Build history of the part. All positions in model axes, mm. Face numbers are marked on the shaded views. A direction names the side the tool comes from. Coordinates: 2 decimals unless noted, no trailing zeros. Order: outer loops, then holes, each group sorted by start corner. A loop starts at its lowest first (then second) coordinate and runs counter-clockwise, first axis right, second up. Notation, with made-up numbers: (78.25, 66) -> (107.25, 66) arc R25 ccw to (107.25, 100) -> close; hole circle Ø7 at (-25.75, -6). An arc over 180 degrees is marked (long way). Write each question's results on one line, items separated by ' | '.
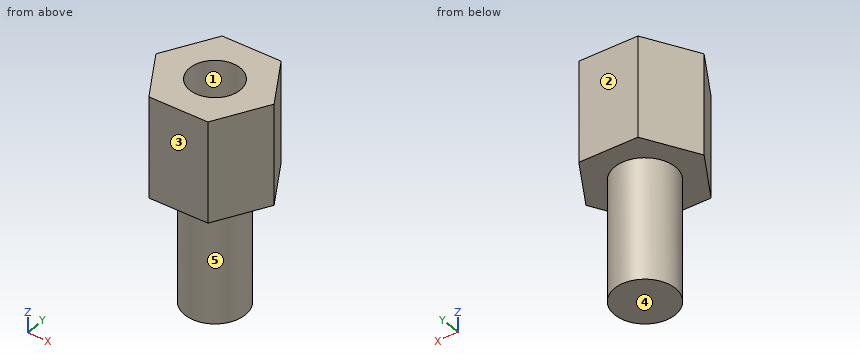
from build123d import *

# Parameters (mm, degrees)
EXTRUDE_1_DEPTH = 5
SKETCH_4_R      = 1.5
EXTRUDE_2_DEPTH = 6
M3X0_5_1_D      = 2.5
M3X0_5_1_DEPTH  = 7.5
M3X0_5_1_TIP    = 0.751075774


with BuildPart() as part:
    # 草圖1 → 填料-伸長1 (new body)
    with BuildSketch(Plane.XY):
        Polygon((-1.443375673, 2.5), (-2.886751346, 0), (-1.443375673, -2.5), (1.443375673, -2.5), (2.886751346, 0), (1.443375673, 2.5), align=None)
    extrude(amount=EXTRUDE_1_DEPTH)

    # 草圖4 → 填料-伸長2 (add)
    with BuildSketch(Plane(origin=(0, 0, 0), x_dir=(-1, 0, 0), z_dir=(0, 0, -1))):
        Circle(SKETCH_4_R)
    extrude(amount=EXTRUDE_2_DEPTH)

    # M3x0.5 螺紋孔1
    with Locations(Plane.XY.offset(5)):
        with Locations((0, 0)):
            Hole(M3X0_5_1_D / 2, depth=M3X0_5_1_DEPTH)
            with Locations((0, 0, -(M3X0_5_1_DEPTH + M3X0_5_1_TIP / 2))):  # 118° drill point
                Cone(0, M3X0_5_1_D / 2, M3X0_5_1_TIP, mode=Mode.SUBTRACT)


solid = part.part
Item 1: Slice it at C-C, the plane y = 2.1. List the corners of the cut face in (x, z).
Answer:
outline: (-1.67, 0) -> (1.67, 0) -> (1.67, 5) -> (-1.67, 5) -> close
Item 2: Slice it at D-D, the plane z = -1.25. List the corners of the cut face in (x, y).
Answer:
outline: circle Ø3 at (0, 0); hole circle Ø2.5 at (0, 0)
Item 3: Pull direction Y, two halves, no side cores. Call the marked faces 1, 2 and 3: released by +Y, released by -Y, zero draft, split by the parting line, or undercut.
Answer:
face 1: undercut | face 2: released by +Y | face 3: released by -Y
Item 4: Drill centre lines: line 1 (Y direction, x = 0, z = 1.75); line 2 (Y direction, x = 0, z = -0.5); line 3 (Z direction, x = 1.4, y = 1.35). Where is each one in solid material? Low to high. Write a range as from..to.
Answer:
line 1: y = -2.5..-1.25, 1.25..2.5 | line 2: y = -1.5..-1.25, 1.25..1.5 | line 3: z = 0..5
Item 5: Tool access for the marked faces 4 and 5: list every direction of +Z, -Z, +X, -X, +Y, -Y with a clear straight run to the whole face (end or side of a thin tool).
Answer:
face 4: -Z, +X, -X, +Y, -Y | face 5: -Z
Item 6: Slice it at A-A, the plane z = 4. List the corners of the cut face in (x, y), and give its area (3 significant figures).
Answer:
outline: (-2.89, 0) -> (-1.44, -2.5) -> (1.44, -2.5) -> (2.89, 0) -> (1.44, 2.5) -> (-1.44, 2.5) -> close; hole circle Ø2.5 at (0, 0) | area: 16.7 mm^2
Item 7: Slice it at B-B, the plane z = -4.5. List the corners of the cut face in (x, y).
Answer:
outline: circle Ø3 at (0, 0)
Item 8: Pin check, flat tips, straight feed: pin 1 (1 mm diameter, centred on x = -1.5, z = -1.5, fed in from -Y); pin 2 (1.5 mm diameter, centred on x = 0.5, z = -4.5, fed in from +Y); pin 3 (2 mm diameter, centred on y = -0.5, z = 3, fed in from -X). Stop position of each tip, or through.
Answer:
pin 1: stops at y = -1.12 | pin 2: stops at y = 1.5 | pin 3: stops at x = -2.89
